Design review of the part built by this model. Coordinates are the model's own, in mm. Coordinates: 2 decimals unless noted, no trailing zeros. Order: outer loops, then holes, each group sorted by start corner. A loop starts at its lowest first (then second) coordinate and runs counter-clockwise, first axis right, second up. Notation, with made-up numbers: M -31,-4.75 L -15,-4.75 A24 cw -15,26.25 Z; hole C -36,-29 d5. An arc over 180 degrees is marked long. Use CSV: the item, a comma, the result in double quotes.
```python
from build123d import *

# Parameters (mm, degrees)
F0_W     = 237
F0_H     = 159
F1_DEPTH = 4
F2_W     = 4
F2_H     = 32
F2_H_2   = 16
F3_DEPTH = 4
F4_W     = 45.8
F4_H     = 4
F5_DEPTH = 4
F6_W     = 47.4
F6_H     = 2
F7_DEPTH = 4


with BuildPart() as f1:
    # F0 (on Top) → F1 (new body)
    with BuildSketch(Plane.XY):
        with Locations((118.5, 79.5)):
            Rectangle(F0_W, F0_H)
    extrude(amount=F1_DEPTH)

    # F2 (on face) → F3 (cut, through all)
    with BuildSketch(Plane.XY.offset(4)):
        with Locations((2, 16)):
            Rectangle(F2_W, F2_H)
        with Locations((2, 71.5)):
            Rectangle(F2_W, F2_H_2)
        with Locations((2, 87.5)):
            Rectangle(F2_W, F2_H_2)
        with Locations((235, 71.5)):
            Rectangle(F2_W, F2_H_2)
        with Locations((235, 87.5)):
            Rectangle(F2_W, F2_H_2)
        with Locations((235, 16)):
            Rectangle(F2_W, F2_H)
        with Locations((235, 143)):
            Rectangle(F2_W, F2_H)
        with Locations((2, 143)):
            Rectangle(F2_W, F2_H)
    extrude(amount=-F3_DEPTH, mode=Mode.SUBTRACT)

    # F4 (on face) → F5 (cut, through all)
    with BuildSketch(Plane.XY.offset(4)):
        with Locations((26.9, 2)):
            Rectangle(F4_W, F4_H)
        with Locations((118.5, 2)):
            Rectangle(F4_W, F4_H)
        with Locations((210.1, 2)):
            Rectangle(F4_W, F4_H)
        with Locations((210.1, 157)):
            Rectangle(F4_W, F4_H)
        with Locations((26.9, 157)):
            Rectangle(F4_W, F4_H)
        with Locations((118.5, 157)):
            Rectangle(F4_W, F4_H)
    extrude(amount=-F5_DEPTH, mode=Mode.SUBTRACT)

    # F6 (on face) → F7 (cut, through all)
    with BuildSketch(Plane.XY.offset(4)):
        with Locations((71.1, 80.5)):
            Rectangle(F6_W, F6_H)
        with Locations((71.1, 78.5)):
            Rectangle(F6_W, F6_H)
        with Locations((165.9, 80.5)):
            Rectangle(F6_W, F6_H)
        with Locations((165.9, 78.5)):
            Rectangle(F6_W, F6_H)
    extrude(amount=-F7_DEPTH, mode=Mode.SUBTRACT)


solid = f1.part
```
(1) Wall thickness on probe 1 along Y at (x, z) = (63, 0.9); probe 2 along Y at (x, z) = (47.5, 0.9); probe 3 along Y at (x, z) = (39, 1.45): over which ranges is each line inside the solid? List them lowest first.
The answers:
probe 1,"y = 0 to 77.5, 81.5 to 159"
probe 2,"y = 4 to 77.5, 81.5 to 155"
probe 3,"y = 4 to 155"
(2) Add section A-A on x = 181.5. State the section outline as (y, z) points.
The answers:
outline,"M 0,0 L 77.5,0 L 77.5,4 L 0,4 Z; M 81.5,0 L 159,0 L 159,4 L 81.5,4 Z"
(3) Add section C-C on y = 13. State the section outline as (x, z) points.
The answers:
outline,"M 4,0 L 233,0 L 233,4 L 4,4 Z"
(4) Clearance check with flat-ended pins moving along their axes: P1, Ø2, axis at y = 78.5, z = 2.5, coming from the +X side; P2, Ø1.2, axis at x = 209.5, z = 1.5, coming from the -Y side; P3, Ø1, axis at y = 130, z = 2, coming from the -X side. State where each tip first meets the part, or that it passes through.
The answers:
P1,"stops at x = 233"
P2,"stops at y = 4"
P3,"stops at x = 4"
(5) Add section D-D on x = 136.5. State the section outline as (y, z) points.
The answers:
outline,"M 4,0 L 155,0 L 155,4 L 4,4 Z"
(6) Add section B-B on z = 1.25. Give the number of separate pieces and of enclosed holes in the cut face, and give its area (3 significant figures).
The answers:
separate pieces,"1"
enclosed holes,"2"
area,"35,400 mm2"
